Can you work these out from the model? Positions are in its coordinate system, mm. A direction names the side the tool comes from. Round coordinates to 2 decimals unless told otherwise and drop trailing zeros. Loops run counter-clockwise (first coordinate to the right, second up) from the corner with the lowest first, then second, coordinate; pieces in that order, holes last. Notation, with made-up numbers: (7, -12.75) - (32, -12.75) arc R25 cw to (32, -0.75) - close; hole circle Ø3 at (-25, 34). An arc over 180 degrees is marked (long way). Answer as CSV lines item,"result".
```python
from build123d import *

# Parameters (mm, degrees)
BOSS_EXTRUDE1_DEPTH   = 25
CUT_EXTRUDE1_DEPTH    = 5
FILLET1_R             = 5
CHAMFER1_SIZE         = 1
M3X0_5_TAPPED_HOLE1_D = 2.5


with BuildPart() as part:
    # Sketch1 → Boss-Extrude1 (new, symmetric)
    with BuildSketch(Plane(origin=(0, 0, 0), x_dir=(0, 0, -1), z_dir=(1, 0, 0))):
        Polygon((-17.5, 10), (17.5, 10), (17.5, 0), (4, 0), (4, -3), (-4, -3), (-4, 0), (-17.5, 0), align=None)
    extrude(amount=BOSS_EXTRUDE1_DEPTH, both=True)

    # Sketch3 → CSK for M6 Flat Head Machine Screw1 (revolve, cut)
    with BuildSketch(Plane(origin=(0, 10, 0), x_dir=(0, 0, 1), z_dir=(1, 0, 0))):
        Polygon((0, 0), (0, 13), (3.3, 13), (3.3, 8), (6.3, 5), (6.3, 0), align=None)
    revolve(axis=Axis((0, 16.35, 0), (0, -1, 0)), mode=Mode.SUBTRACT)

    # Sketch4 → Cut-Extrude1 (cut, symmetric)
    with BuildSketch(Plane(origin=(15, 0, 0), x_dir=(0, 0, -1), z_dir=(1, 0, 0))):
        with BuildLine():
            Line((-15, 10), (-10, 10))
            ThreePointArc((-10, 10), (-7.5, 7.5), (-5, 10))
            Line((-5, 10), (0, 10))
            ThreePointArc((0, 10), (-7.5, 2.5), (-15, 10))
        make_face()
    cut_extrude1 = extrude(amount=CUT_EXTRUDE1_DEPTH, both=True, mode=Mode.SUBTRACT)

    # Mirror1: Cut-Extrude1 across plane
    add(cut_extrude1.mirror(Plane(origin=(0, 0, 0), x_dir=(0, 0, 1), z_dir=(1, 0, 0))), mode=Mode.SUBTRACT)

    # Fillet1
    fillet1_edges = [part.edges().sort_by_distance(p)[0] for p in [
        (-25, 5, 17.5),
        (25, 5, -17.5),
        (25, 5, 17.5),
        (-25, 5, -17.5),
    ]]
    fillet(fillet1_edges, radius=FILLET1_R)

    # Chamfer1
    # the kernel refuses this chamfer: 1 mm, written as the material it takes off along each edge
    with BuildSketch(Plane(origin=(-25, -5.571682988, 4), x_dir=(-0.027495876610585623, 0, -0.9996219169112968), z_dir=(0, 1, 0)), Plane(origin=(-25, 0, -4), x_dir=(-0.027495876610585623, 0, 0.9996219169112968), z_dir=(0, -1, 0))) as chamfer1_piece_1:
        Polygon((CHAMFER1_SIZE * 0.999621916911, -CHAMFER1_SIZE * 0.0274958766106), (-CHAMFER1_SIZE * 0.0274958766106, -CHAMFER1_SIZE * 0.999621916911), (0, 0), align=None)
    extrude(amount=5.571682988, mode=Mode.SUBTRACT)
    with BuildSketch(Plane(origin=(25, -5.571682988, 4), x_dir=(0.027495876610585623, 0, -0.9996219169112968), z_dir=(0, 1, 0)), Plane(origin=(25, 0, -4), x_dir=(0.027495876610585623, 0, 0.9996219169112968), z_dir=(0, -1, 0))) as chamfer1_piece_2:
        Polygon((CHAMFER1_SIZE * 0.999621916911, CHAMFER1_SIZE * 0.0274958766106), (-CHAMFER1_SIZE * 0.0274958766106, CHAMFER1_SIZE * 0.999621916911), (0, 0), align=None)
    extrude(amount=5.571682988, mode=Mode.SUBTRACT)
    with BuildSketch(Plane(origin=(27.571682988, -3, -4), x_dir=(0, 0.9996219169112968, -0.027495876610586494), z_dir=(-1, 0, 0))) as chamfer1_piece_3:
        Polygon((CHAMFER1_SIZE * 0.999621916911, -CHAMFER1_SIZE * 0.0274958766106), (-CHAMFER1_SIZE * 0.0274958766106, -CHAMFER1_SIZE * 0.999621916911), (0, 0), align=None)
    extrude(amount=55.143365976, mode=Mode.SUBTRACT)
    with BuildSketch(Plane(origin=(27.571682988, -3, 4), x_dir=(0, 0.9996219169112968, 0.027495876610586494), z_dir=(-1, 0, 0))) as chamfer1_piece_4:
        Polygon((CHAMFER1_SIZE * 0.999621916911, CHAMFER1_SIZE * 0.0274958766106), (-CHAMFER1_SIZE * 0.0274958766106, CHAMFER1_SIZE * 0.999621916911), (0, 0), align=None)
    extrude(amount=55.143365976, mode=Mode.SUBTRACT)
    with BuildSketch(Plane(origin=(25, 0, -12.5), x_dir=(0.027495876610585623, 0.9996219169112968, 0), z_dir=(0, 0, 1)), Plane(origin=(25, 0, 4), x_dir=(0.02749587661058563, 0.9996219169112968, 0), z_dir=(0, 0, 1))) as chamfer1_piece_5:
        Polygon((CHAMFER1_SIZE * 0.999621916911, CHAMFER1_SIZE * 0.0274958766106), (-CHAMFER1_SIZE * 0.0274958766106, CHAMFER1_SIZE * 0.999621916911), (0, 0), align=None)
    extrude(amount=8.5, mode=Mode.SUBTRACT)
    with BuildSketch(Plane(origin=(-25, 0, 4), x_dir=(-0.02749587661058563, 0.9996219169112968, 0), z_dir=(0, 0, 1)), Plane(origin=(-25, 0, -12.5), x_dir=(-0.027495876610585623, 0.9996219169112968, 0), z_dir=(0, 0, 1))) as chamfer1_piece_6:
        Polygon((CHAMFER1_SIZE * 0.999621916911, -CHAMFER1_SIZE * 0.0274958766106), (-CHAMFER1_SIZE * 0.0274958766106, -CHAMFER1_SIZE * 0.999621916911), (0, 0), align=None)
    extrude(amount=8.5, mode=Mode.SUBTRACT)
    with BuildSketch(Plane(origin=(-20, 0, 17.5), x_dir=(0, 0.9996219169112968, 0.02749587661058563), z_dir=(1, 0, 0)), Plane(origin=(20, 0, -17.5), x_dir=(0, 0.9996219169112968, -0.027495876610585623), z_dir=(-1, 0, 0))) as chamfer1_piece_7:
        Polygon((CHAMFER1_SIZE * 0.999621916911, -CHAMFER1_SIZE * 0.0274958766106), (-CHAMFER1_SIZE * 0.0274958766106, -CHAMFER1_SIZE * 0.999621916911), (0, 0), align=None)
    extrude(amount=40, mode=Mode.SUBTRACT)
    with BuildSketch(Plane(origin=(-20, 0, 12.5), x_dir=(0, 0, 1), z_dir=(1, 0, 0))) as chamfer1_piece_8:
        Polygon((5, -CHAMFER1_SIZE), (5 - CHAMFER1_SIZE, 0), (5, 0), align=None)
    revolve(axis=Axis((-20, 0, 12.5), (0, -1, 0)), revolution_arc=90, mode=Mode.SUBTRACT)
    with BuildSketch(Plane(origin=(20, 0, 12.5), x_dir=(0, 0, 1), z_dir=(-1, 0, 0))) as chamfer1_piece_9:
        Polygon((5, CHAMFER1_SIZE), (5 - CHAMFER1_SIZE, 0), (5, 0), align=None)
    revolve(axis=Axis((20, 0, 12.5), (0, 1, 0)), revolution_arc=90, mode=Mode.SUBTRACT)
    with BuildSketch(Plane(origin=(-20, 0, -12.5), x_dir=(-1, 0, 0), z_dir=(0, 0, 1))) as chamfer1_piece_10:
        Polygon((5, -CHAMFER1_SIZE), (5 - CHAMFER1_SIZE, 0), (5, 0), align=None)
    revolve(axis=Axis((-20, 0, -12.5), (0, -1, 0)), revolution_arc=90, mode=Mode.SUBTRACT)
    with BuildSketch(Plane(origin=(20, 0, -12.5), x_dir=(1, 0, 0), z_dir=(0, 0, 1))) as chamfer1_piece_11:
        Polygon((5, CHAMFER1_SIZE), (5 - CHAMFER1_SIZE, 0), (5, 0), align=None)
    revolve(axis=Axis((20, 0, -12.5), (0, 1, 0)), revolution_arc=90, mode=Mode.SUBTRACT)
    with BuildSketch(Plane(origin=(-25, 0, 1.428317012), x_dir=(-0.02749587661058563, 0.9996219169112968, 0), z_dir=(0, 0, 1))) as chamfer1_piece_12a_section:
        Polygon((CHAMFER1_SIZE * 0.999621916911, -CHAMFER1_SIZE * 0.0274958766106), (-CHAMFER1_SIZE * 0.0274958766106, -CHAMFER1_SIZE * 0.999621916911), (0, 0), align=None)
    chamfer1_piece_12a = extrude(amount=11.071682988, mode=Mode.PRIVATE)
    chamfer1_piece_12a = split(chamfer1_piece_12a, bisect_by=Plane(origin=(-24.670206373, 0.329793627, 4), z_dir=(0, 0, -1)), keep=Keep.TOP, mode=Mode.PRIVATE)
    with BuildSketch(Plane(origin=(-25, -5.571682988, 4), x_dir=(-0.027495876610585623, 0, -0.9996219169112968), z_dir=(0, 1, 0))) as chamfer1_piece_12b_section:
        Polygon((CHAMFER1_SIZE * 0.999621916911, -CHAMFER1_SIZE * 0.0274958766106), (-CHAMFER1_SIZE * 0.0274958766106, -CHAMFER1_SIZE * 0.999621916911), (0, 0), align=None)
    chamfer1_piece_12b = extrude(amount=8.143365976, mode=Mode.PRIVATE)
    chamfer1_piece_12b = split(chamfer1_piece_12b, bisect_by=Plane(origin=(-24.670206373, 0, 3.670206373), z_dir=(0, 1, 0)), keep=Keep.TOP, mode=Mode.PRIVATE)
    chamfer1_piece_12 = chamfer1_piece_12a & chamfer1_piece_12b
    add(chamfer1_piece_12, mode=Mode.SUBTRACT)
    with BuildSketch(Plane(origin=(25, 0, 1.428317012), x_dir=(0.02749587661058563, 0.9996219169112968, 0), z_dir=(0, 0, 1))) as chamfer1_piece_13a_section:
        Polygon((CHAMFER1_SIZE * 0.999621916911, CHAMFER1_SIZE * 0.0274958766106), (-CHAMFER1_SIZE * 0.0274958766106, CHAMFER1_SIZE * 0.999621916911), (0, 0), align=None)
    chamfer1_piece_13a = extrude(amount=11.071682988, mode=Mode.PRIVATE)
    chamfer1_piece_13a = split(chamfer1_piece_13a, bisect_by=Plane(origin=(24.670206373, 0.329793627, 4), z_dir=(0, 0, -1)), keep=Keep.TOP, mode=Mode.PRIVATE)
    with BuildSketch(Plane(origin=(25, -5.571682988, 4), x_dir=(0.027495876610585623, 0, -0.9996219169112968), z_dir=(0, 1, 0))) as chamfer1_piece_13b_section:
        Polygon((CHAMFER1_SIZE * 0.999621916911, CHAMFER1_SIZE * 0.0274958766106), (-CHAMFER1_SIZE * 0.0274958766106, CHAMFER1_SIZE * 0.999621916911), (0, 0), align=None)
    chamfer1_piece_13b = extrude(amount=8.143365976, mode=Mode.PRIVATE)
    chamfer1_piece_13b = split(chamfer1_piece_13b, bisect_by=Plane(origin=(24.670206373, 0, 3.670206373), z_dir=(0, 1, 0)), keep=Keep.TOP, mode=Mode.PRIVATE)
    chamfer1_piece_13 = chamfer1_piece_13a & chamfer1_piece_13b
    add(chamfer1_piece_13, mode=Mode.SUBTRACT)
    with BuildSketch(Plane(origin=(25, 0, -12.5), x_dir=(0.027495876610585623, 0.9996219169112968, 0), z_dir=(0, 0, 1))) as chamfer1_piece_14a_section:
        Polygon((CHAMFER1_SIZE * 0.999621916911, CHAMFER1_SIZE * 0.0274958766106), (-CHAMFER1_SIZE * 0.0274958766106, CHAMFER1_SIZE * 0.999621916911), (0, 0), align=None)
    chamfer1_piece_14a = extrude(amount=11.071682988, mode=Mode.PRIVATE)
    chamfer1_piece_14a = split(chamfer1_piece_14a, bisect_by=Plane(origin=(24.670206373, 0.329793627, -4), z_dir=(0, 0, 1)), keep=Keep.TOP, mode=Mode.PRIVATE)
    with BuildSketch(Plane(origin=(25, 2.571682988, -4), x_dir=(0.027495876610585623, 0, 0.9996219169112968), z_dir=(0, -1, 0))) as chamfer1_piece_14b_section:
        Polygon((CHAMFER1_SIZE * 0.999621916911, CHAMFER1_SIZE * 0.0274958766106), (-CHAMFER1_SIZE * 0.0274958766106, CHAMFER1_SIZE * 0.999621916911), (0, 0), align=None)
    chamfer1_piece_14b = extrude(amount=8.143365976, mode=Mode.PRIVATE)
    chamfer1_piece_14b = split(chamfer1_piece_14b, bisect_by=Plane(origin=(24.670206373, 0, -3.670206373), z_dir=(0, 1, 0)), keep=Keep.TOP, mode=Mode.PRIVATE)
    chamfer1_piece_14 = chamfer1_piece_14a & chamfer1_piece_14b
    add(chamfer1_piece_14, mode=Mode.SUBTRACT)
    with BuildSketch(Plane(origin=(-25, 0, -12.5), x_dir=(-0.027495876610585623, 0.9996219169112968, 0), z_dir=(0, 0, 1))) as chamfer1_piece_15a_section:
        Polygon((CHAMFER1_SIZE * 0.999621916911, -CHAMFER1_SIZE * 0.0274958766106), (-CHAMFER1_SIZE * 0.0274958766106, -CHAMFER1_SIZE * 0.999621916911), (0, 0), align=None)
    chamfer1_piece_15a = extrude(amount=11.071682988, mode=Mode.PRIVATE)
    chamfer1_piece_15a = split(chamfer1_piece_15a, bisect_by=Plane(origin=(-24.670206373, 0.329793627, -4), z_dir=(0, 0, 1)), keep=Keep.TOP, mode=Mode.PRIVATE)
    with BuildSketch(Plane(origin=(-25, 2.571682988, -4), x_dir=(-0.027495876610585623, 0, 0.9996219169112968), z_dir=(0, -1, 0))) as chamfer1_piece_15b_section:
        Polygon((CHAMFER1_SIZE * 0.999621916911, -CHAMFER1_SIZE * 0.0274958766106), (-CHAMFER1_SIZE * 0.0274958766106, -CHAMFER1_SIZE * 0.999621916911), (0, 0), align=None)
    chamfer1_piece_15b = extrude(amount=8.143365976, mode=Mode.PRIVATE)
    chamfer1_piece_15b = split(chamfer1_piece_15b, bisect_by=Plane(origin=(-24.670206373, 0, -3.670206373), z_dir=(0, 1, 0)), keep=Keep.TOP, mode=Mode.PRIVATE)
    chamfer1_piece_15 = chamfer1_piece_15a & chamfer1_piece_15b
    add(chamfer1_piece_15, mode=Mode.SUBTRACT)

    # M3x0.5 Tapped Hole1 (through all)
    with Locations(Plane(origin=(0, 10, 0), x_dir=(1, 0, 0), z_dir=(0, 1, 0))):
        with Locations((-9.5, 13), (9.5, 13)):
            Hole(M3X0_5_TAPPED_HOLE1_D / 2)


solid = part.part
```
Q1. Imagine slicing it at D-D (z = -7). Write out the boundary of the cut face in (x, y).
Checks:
outline,"(-25, 1) - (-24, 0) - (24, 0) - (25, 1) - (25, 10) - (-25, 10) - close"
Q2. I'm going to push flat-ended pins straight in: pin 1 Ø10 at (x, z) = (-4.5, -8.5) entering from -Y; pin 2 Ø0.6 at (x, y) = (-7, -0.5) entering from +Z; pin 3 Ø1 at (x, y) = (6.5, -1) entering from -Z. Where does each tip first touch, or does it pass through?
Checks:
pin 1,"y = -2.5"
pin 2,"z = 4"
pin 3,"z = -4"
Q3. We'd pull the mould along X, two halves only. Please class faces 5 (the flat face through (-24.5, 0.5, 7.7)), 6 (the flat face through (24.5, 0.5, 7.7)), 7 (the flat face through (-20, 6, 7)): pulls with the +X half, pulls with the -X half, needs draft (parallel to the pull), parting line crosses it, or undercut.
Checks:
face 5,"pulls with the -X half"
face 6,"pulls with the +X half"
face 7,"undercut"
Q4. If I drill on line 1 along X through (y, z) = (8, -13); line 2 along X through (y, z) = (3.5, 6.5); line 3 along Z through (x, y) = (-9.5, 6), over which ranges is the centre line in solid material (lowest first)? Write a range as [from, to].
Checks:
line 1,"[-24.97, -10.75], [-8.25, 8.25], [10.75, 24.97]"
line 2,"[-25, -20], [-10, 10], [20, 25]"
line 3,"[-17.5, -14.25], [-11.75, 17.5]"
Q5. Imagine slicing it at C-C (x = 0). Write out the boundary of the cut face in (y, z).
Checks:
outline,"(-2.7, -3.3) - (-2, -4) - (0, -4) - (0, -16.5) - (1, -17.5) - (10, -17.5) - (10, -6.3) - (5, -6.3) - (2, -3.3) - close; (-2.7, 3.3) - (2, 3.3) - (5, 6.3) - (10, 6.3) - (10, 17.5) - (1, 17.5) - (0, 16.5) - (0, 4) - (-2, 4) - close"
Q6. On a 3-axis mill with a long thin cutter (end or side, diameter ignored), from which of +Z, -Z, +X, -X, +Y, -Y can I reach the whole of each face in a straight line? I mean faces 1 (the cylindrical face through (10.421, 4.93, -13.845)), 2 (the cylindrical face through (15.1, 7.5, 7.6)), 3 (the flat face through (-24.6, -1, -3.4)), 4 (the flat face through (0, 0, 10)). Say none if no direction works.
Checks:
face 1,"+Y, -Y"
face 2,"none"
face 3,"-Z, -X, -Y"
face 4,"+Z, +X, -X, -Y"
Q7. Imagine slicing it at A-A (x = -9.5). Write out the boundary of the cut face in (y, z), then the cut area to 3 significant figures.
Checks:
outline,"(-3, -3) - (-2, -4) - (0, -4) - (0, -11.75) - (10, -11.75) - (10, 17.5) - (1, 17.5) - (0, 16.5) - (0, 4) - (-2, 4) - (-3, 3) - close; (0, -16.5) - (1, -17.5) - (10, -17.5) - (10, -14.25) - (0, -14.25) - close"
area,"347 mm²"
Q8. Imagine slicing it at B-B (z = 7.5). Write out the boundary of the cut face in (x, y).
Checks:
outline,"(-25, 1) - (-24, 0) - (24, 0) - (25, 1) - (25, 10) - (-25, 10) - close; hole (-20, 2.5) - (-10, 2.5) - (-10, 7.5) - (-20, 7.5) - close; hole (10, 2.5) - (20, 2.5) - (20, 7.5) - (10, 7.5) - close"
